Autodesk Inventor part; units mm, degrees
ref_plane "YZ Plane" through (0, 0, 0) normal (1, 0, 0) x (0, 1, 0)
ref_plane "XZ Plane" through (0, 0, 0) normal (0, 1, 0) x (-1, 0, 0)
ref_plane "XY Plane" through (0, 0, 0) normal (0, 0, 1) x (1, 0, 0)
sketch "Sketch1" plane through (0, 0, 0) normal (1, 0, 0) x (0, 1, 0)
  line L0 (0, 3) -> (14, 3)
  line L1 (14, 3) -> (14, -2)
  line L2 (14, -2) -> (0, -2)
  line L3 (0, -2) -> (0, 3)
  line L4 (0, -3) -> (0, 4)
  line L5 (14, 1.5) -> (14, -0.5)
  line L6 (14, -0.5) -> (10, -0.5)
  line L7 (10, -0.5) -> (10, 1.5)
  line L8 (10, 1.5) -> (14, 1.5)
  point P0 (0, 0)
  dimension "d0" = 5
  dimension "d1" = 3
  dimension "d2" = 14
  dimension "d4" = 1.5
  dimension "d5" = 1.5
  dimension "d19" = 4
revolve "Revolution1" add sketch "Sketch1" angle 360 about axis through (0, 0, -10) along (0, 0, 1) contours L0 L1 L8 L7 L6 L2 L3
sketch "Sketch2" plane through (0, 0, -2) normal (0, 0, -1) x (-1, 0, 0)
  circle A0 centre (0, 8) radius 1.05
  circle A1 centre (0, 0) radius 4.5
  dimension "d7" = 2.1
  dimension "d8" = 8
  dimension "d9" = 9
extrude "Extrusion1" cut sketch "Sketch2" against normal blind 100
pattern_circular "Circular Pattern1" count 8 over 360 about axis through (0, 0, -10) along (0, 0, 1) of "Extrusion1"
sketch "Sketch3" plane through (0, 0, -2) normal (0, 0, -1) x (-1, 0, 0)
  circle A0 centre (-10.5, 0) radius 1
  point P0 (0, 0)
  dimension "d15" = 2
  dimension "d16" = 10.5
extrude "Extrusion2" cut sketch "Sketch3" against normal blind 100
sketch "Sketch4" plane through (0, 0, -2) normal (0, 0, -1) x (-1, 0, 0)
  circle A0 centre (-10.5, 0) radius 1
  circle A1 centre (-8, 0) radius 1.05
  circle A2 centre (0, -8) radius 1.05
  circle A3 centre (8, 0) radius 1.05
  circle A4 centre (5.6569, 5.6569) radius 1.05
  circle A5 centre (5.6569, -5.6569) radius 1.05
  circle A6 centre (-5.6569, -5.6569) radius 1.05
  circle A7 centre (-5.6569, 5.6569) radius 1.05
  circle A8 centre (0, 0) radius 4.5
  circle A9 centre (0, 8) radius 1.05
  circle A10 centre (0, 0) radius 14
  arc A11 (-9.9643, -0.8444) -> (-9.9643, 0.8444) centre (0, 0) ccw
  arc A12 (-9.9643, -0.8444) -> (-9.9643, 0.8444) centre (0, 0) ccw
  circle A13 centre (0, 0) radius 5.125
  point P0 (-9.9643, -0.8444)
  point P1 (-9.9643, 0.8444)
  dimension "d24" = 10.25
extrude "Extrusion3" add sketch "Sketch4" along normal blind 5 and the other way blind 2 contours A8 | A13
sketch "Sketch9" plane through (0, 0, 0) normal (0, 0, 1) x (1, 0, 0)
  circle A0 centre (0, 0) radius 2.5
  dimension "d37" = 5
extrude "Extrusion8" cut sketch "Sketch9" against normal blind 1
sketch "Sketch7" plane through (0, 0, -7) normal (0, 0, -1) x (-1, 0, 0)
  circle A0 centre (-5.125, 0) radius 1
  circle A1 centre (0, 0) radius 5.125
  dimension "d31" = 2
extrude "Extrusion6" cut sketch "Sketch7" against normal blind 4 contours A0 A1 | A1 A0 picked at (-4.7844, 0) picked at (-5.4511, 0)
sketch "Sketch8" plane through (0, 0, -7) normal (0, 0, -1) x (-1, 0, 0)
  circle A0 centre (0, 0) radius 9
  arc A1 (-5.0274, -0.9952) -> (-5.0274, 0.9952) centre (-5.125, 0) ccw
  arc A2 (-5.0274, -0.9952) -> (-5.0274, 0.9952) centre (-5.125, 0) ccw
  circle A3 centre (-5.125, 0) radius 1
  arc A4 (-5.0274, -0.9952) -> (-5.0274, 0.9952) centre (0, 0) ccw
  point P0 (-4.3889, 0.9938)
  point P1 (-4.3889, -0.9938)
  point P2 (-5.0274, -0.9952)
  point P3 (-5.0274, 0.9952)
  dimension "d34" = 18
extrude "Extrusion7" add sketch "Sketch8" along normal blind 1.5 contours A0 | A1 A4
sketch "Sketch11" plane through (0, 0, -2) normal (0, 0, -1) x (-1, 0, 0)
  circle A0 centre (-10.5, 0) radius 1
  circle A1 centre (-8, 0) radius 1.05
  circle A2 centre (0, -8) radius 1.05
  circle A3 centre (8, 0) radius 1.05
  circle A4 centre (5.6569, 5.6569) radius 1.05
  circle A5 centre (5.6569, -5.6569) radius 1.05
  circle A6 centre (-5.6569, -5.6569) radius 1.05
  circle A7 centre (-5.6569, 5.6569) radius 1.05
  circle A8 centre (0, 8) radius 1.05
  circle A9 centre (0, 0) radius 14
  circle A10 centre (-5.6569, 5.6569) radius 2
  circle A11 centre (0, 8) radius 2
  circle A12 centre (5.6569, 5.6569) radius 2
  circle A13 centre (8, 0) radius 2
  circle A14 centre (5.6569, -5.6569) radius 2
  circle A15 centre (0, -8) radius 2
  circle A16 centre (-5.6569, -5.6569) radius 2
  line L0 (-7.5, 3) -> (-18.9706, 3)
  line L1 (-18.9706, 3) -> (-18.9706, -3)
  line L2 (-18.9706, -3) -> (-7.5, -3)
  line L3 (-7.5, -3) -> (-7.5, 3)
  circle A17 centre (0, 0) radius 5.125
  point P0 (-4.3889, -0.9938)
  point P1 (-4.3889, 0.9938)
  point P2 (-7.5, -0.9233)
  point P3 (-13.6748, -3)
  point P4 (-13.6748, 3)
  point P5 (-7.5, 0.9233)
  dimension "d44" = 4
  dimension "d45" = 4
  dimension "d46" = 4
  dimension "d47" = 4
  dimension "d48" = 4
  dimension "d49" = 4
  dimension "d50" = 4
  dimension "d51" = 3
  dimension "d52" = 3
  dimension "d53" = 3
extrude "Extrusion10" add sketch "Sketch11" along normal blind 1.6 contours A1 L3 L0 A9 L2 | A17 picked at (-11.2403, -4.0708)
extrude "Extrusion11" add sketch "Sketch11" against normal blind 6 contours A1 L3 | L3 A1
sketch "Sketch10" plane through (0, 0, -7) normal (0, 0, 1) x (1, 0, 0)
  circle A0 centre (0, 0) radius 24.9442
extrude "Extrusion9" cut sketch "Sketch10" against normal blind 100
properties part number "Motor_pulley_p2"
Geometry: final body of the model. Coordinates: model frame, mm. A direction names the side the tool comes from. Round coordinates to 2 decimals unless told otherwise and drop trailing zeros. Write each loop counter-clockwise with the first axis right and the second up, starting at its lowest first coordinate (ties: lowest second). Pieces come first, ordered by that corner, then holes.
Item 1: Pin query (flat end, axial travel): P1, Ø6, axis at y = 5, z = 2, coming from the -X side; P2, Ø1.8, axis at y = 2.5, z = -3, coming from the +X side; P3, Ø5, axis at y = -10, z = 1, coming from the +X side. Return the tip coordinate at first contact, or that it passes through.
Item 2: Section query B-B (x = -8). Return loops of the section in (y, z), plus the area to 3 significant figures.
Item 3: Section query A-A (y = 11.25). Return loops of the section in (x, z), plus the area to 3 significant figures.
Item 4: Material intervals for L1, parallel to Y at x = 0, z = -2.95; L2, parallel to Z at x = -9.25, y = 5.75; L3, parallel to Z at x = 12, y = 0, sorted ascending.
Item 5: Mould query, pull axis Y, two halves, no side actions, for faces 4 (the face through (-5.362, 12.932, 2.24)), 5 (the face through (-10, -3, 1.5)), 6 (the face through (0, -10, -3)). Classes: +Y half, -Y half, draft (parallel to the pull), parting line (faces both ways), or undercut.
Item 6: Section query D-D (x = 0). Give the number of separate pieces and of enclosed holes in the cut face, plus the area to 3 significant figures.
Item 7: Set-up query: faces 1 (the face through (11, -3, -3)), 2 (the face through (0.56, -8.89, 0.46)), 3 (the face through (7, -5, -2)). Return all of +Z, -Z, +X, -X, +Y, -Y with unobstructed straight access to the full face (end or side cutting, diameter ignored); none if empty.
Completed:
1. P1: stops at x = -13.86
1. P2: stops at x = 13.67
1. P3: stops at x = 11.79
2. outline: (-11.49, -3.6) - (-2, -3.6) - (-2, -2) - (-1.05, -2) - (-1.05, 3) - (-11.49, 3) - (-11.49, 1.5) - (-6, 1.5) - (-6, -0.5) - (-11.49, -0.5) - close; (1.05, -2) - (2, -2) - (2, -3.6) - (11.49, -3.6) - (11.49, -0.5) - (6, -0.5) - (6, 1.5) - (11.49, 1.5) - (11.49, 3) - (1.05, 3) - close
2. area: 113 mm2
3. outline: (-8.33, -3.6) - (8.33, -3.6) - (8.33, -0.5) - (-8.33, -0.5) - close; (-8.33, 1.5) - (8.33, 1.5) - (8.33, 3) - (-8.33, 3) - close
3. area: 76.7 mm2
4. L1: y = -14 to -10, -6 to 6, 10 to 14
4. L2: z = -3.6 to -0.5, 1.5 to 3
4. L3: z = -2 to -0.5, 1.5 to 3
5. face 4: parting line
5. face 5: draft
5. face 6: undercut
6. separate pieces: 3
6. enclosed holes: 0
6. area: 138 mm2
7. face 1: -Z, +X
7. face 2: +Z, -Z
7. face 3: -Z
